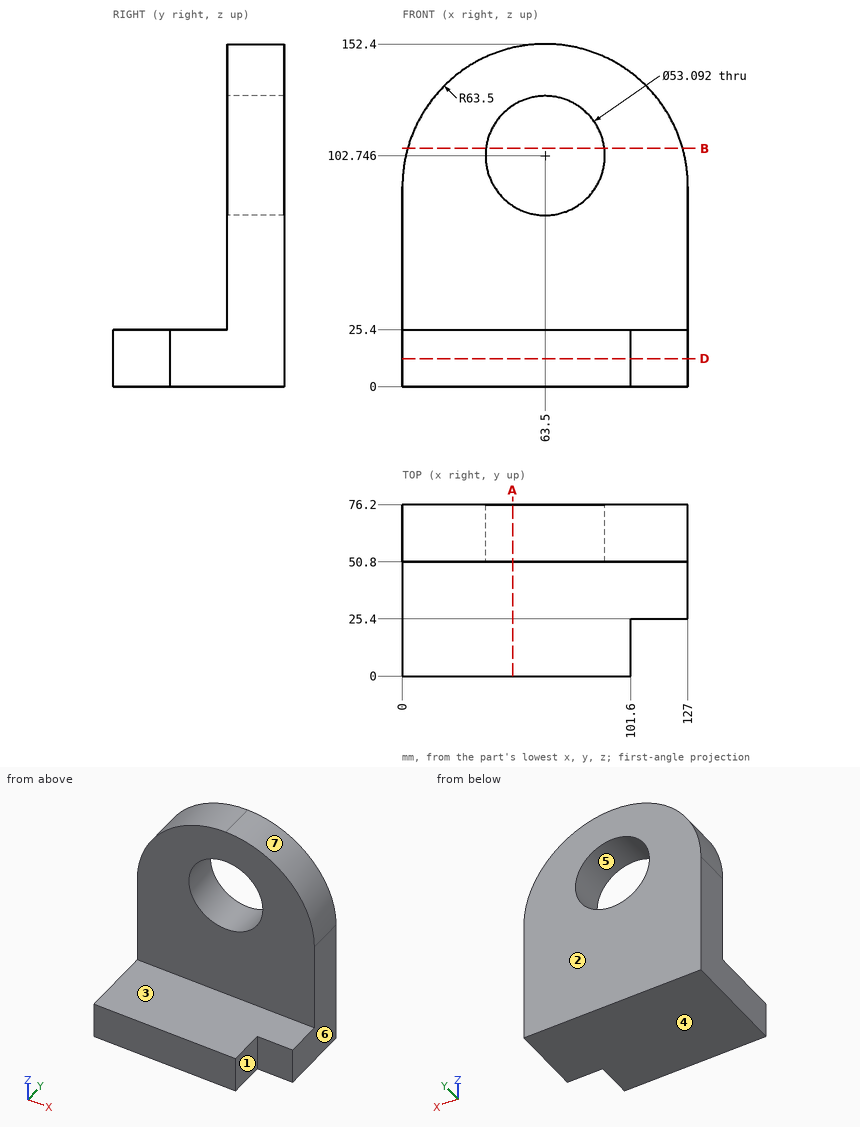
Can you work these out from the drawing? Everything is in mm from the part's minimum corner. A direction names the side the tool comes from. Give positions to 0.01 mm unless a question says otherwise; leave off trailing zeros. Loops run counter-clockwise (first coordinate to the right, second up) from the corner with the lowest first, then second, coordinate; pieces in that order, holes last. Notation, with made-up numbers: (19, 47.25) -> (65, 47.25) arc R13 ccw to (65, 62.25) -> close; hole circle Ø3 at (69, 51). An arc over 180 degrees is marked (long way). Write item = value, one per line.
1) I need wall thicknesses on L1, parallel to Y at x = 38, z = 29; L2, parallel to Z at x = 14, y = 22; L3, parallel to X at y = 68, z = 117 (1 decimal). Which ranges of each line are inside material? Lowest first, please. Write a range as from..to.
Check result:
L1 = 50.8..76.2
L2 = 0..25.4
L3 = 6.6..41.1, 85.9..120.4
2) Suppose I cut it at A-A on x = 49. Write out the boundary of the cut face in (y, z).
Check result:
outline = (0, 0) -> (76.2, 0) -> (76.2, 80.51) -> (50.8, 80.51) -> (50.8, 25.4) -> (0, 25.4) -> close; (50.8, 124.98) -> (76.2, 124.98) -> (76.2, 150.72) -> (50.8, 150.72) -> close
3) Suppose I cut it at B-B on z = 106. Write out the boundary of the cut face in (x, y).
Check result:
outline = (2.35, 50.8) -> (37.15, 50.8) -> (37.15, 76.2) -> (2.35, 76.2) -> close; (89.85, 50.8) -> (124.65, 50.8) -> (124.65, 76.2) -> (89.85, 76.2) -> close
4) Will these pins go through, and if not, where does the flat tip stop? pin 1 (6 mm diameter, centred on x = 27.5, y = 63, fed in from +Z); pin 2 (1.5 mm diameter, centred on x = 49, y = 20.5, fed in from +Z); pin 3 (12 mm diameter, centred on x = 42, z = 104.5, fed in from -Y).
Check result:
pin_1 = 143.15
pin_2 = 25.4
pin_3 = 50.8
5) Thinking about a two-plate mould opening in Z: for the marked faces 4, 5, 6 and 7, which applies, released by +Z, released by -Z, zero draft, split by the parting line, or undercut?
Check result:
face_4 = released by -Z
face_5 = undercut
face_6 = zero draft
face_7 = released by +Z
6) For the marked faces 1, 2 and 3, which set-ups out of +Z, -Z, +X, -X, +Y, -Y let a thin tool reach every point of the face, with its end or its side?
Check result:
face_1 = +Z, -Z, +X, -Y
face_2 = +Z, -Z, +X, -X, +Y
face_3 = +Z, +X, -X, -Y
7) Suppose I cut it at D-D on z = 12.5. Write out the boundary of the cut face in (x, y), then the cut area to 3 significant figures.
Check result:
outline = (0, 0) -> (101.6, 0) -> (101.6, 25.4) -> (127, 25.4) -> (127, 76.2) -> (0, 76.2) -> close
area = 9,030 mm2
